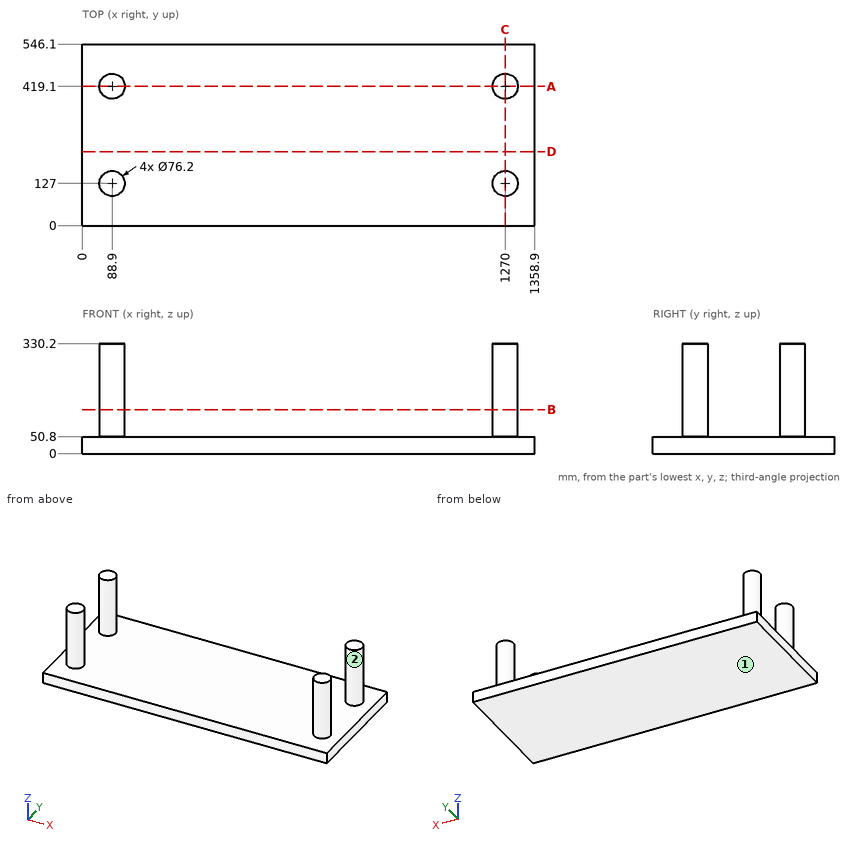
Design review of the part shown in the three views and the two pictorial views. Dimensions are in mm from the part's minimum x, y and z. Give positions to 0.01 mm unless a question says otherwise; leave off trailing zeros. Loops run counter-clockwise (first coordinate to the right, second up) from the corner with the lowest first, then second, coordinate; pieces in that order, holes last. Notation, with made-up numbers: M -32,2 L 13,2 A36 cw 13,36 Z; hole C 24.5,83 d10. An arc over 180 degrees is marked long. Put each result on its own line as item: value. Start each with the question number.
(1) Add section D-D, the plane y = 222.5. Write out the cut boundary in (x, z), then the cut area to 3 significant figures.
(2) The part is to be moulded in two halves that separate along Y. For the marked faces 1 and 2, say which applies: +Y half, -Y half, draft (parallel to the pull), parting line (faces both ways), or undercut.
(3) Add section B-B, the plane z = 132. Write out the cut boundary in (x, y), then the cut area to 3 significant figures.
(4) Wall thickness on L1, parallel to Z at x = 1212, y = 163.5; L2, parallel to X at y = 139.5, z = 282.5; L3, parallel to X at y = 117, z = 111.5: over which ranges is each line inside the solid? List them lowest first.
(5) Add section A-A, the plane y = 419.1. Write out the cut boundary in (x, z), then the cut area to 3 significant figures.
(6) For pin 1 (5 mm diameter, centred on x = 679.5, y = 318, fed in from +Z); pin 2 (12 mm diameter, centred on y = 419.5, z = 220.5, fed in from -X); pin 3 (5 mm diameter, centred on x = 1066, y = 383, fed in from -Z), all flat-tipped, find the tip position at first contact; note any pin that passes through.
(7) Add section C-C, the plane x = 1270. Write out the cut boundary in (y, z), then the cut area to 3 significant figures.
Result:
1. outline: M 0,0 L 1358.9,0 L 1358.9,50.8 L 0,50.8 Z
1. area: 69,000 mm^2
2. face 1: draft
2. face 2: undercut
3. outline: C 88.9,127 d76.2; C 88.9,419.1 d76.2; C 1270,127 d76.2; C 1270,419.1 d76.2
3. area: 18,200 mm^2
4. L1: z = 0 to 50.8
4. L2: x = 52.91 to 124.89, 1234.01 to 1305.99
4. L3: x = 52.14 to 125.66, 1233.24 to 1306.76
5. outline: M 0,0 L 1358.9,0 L 1358.9,50.8 L 1308.1,50.8 L 1308.1,330.2 L 1231.9,330.2 L 1231.9,50.8 L 127,50.8 L 127,330.2 L 50.8,330.2 L 50.8,50.8 L 0,50.8 Z
5. area: 112,000 mm^2
6. pin 1: stops at z = 50.8
6. pin 2: stops at x = 50.8
6. pin 3: stops at z = 0
7. outline: M 0,0 L 546.1,0 L 546.1,50.8 L 457.2,50.8 L 457.2,330.2 L 381,330.2 L 381,50.8 L 165.1,50.8 L 165.1,330.2 L 88.9,330.2 L 88.9,50.8 L 0,50.8 Z
7. area: 70,300 mm^2
